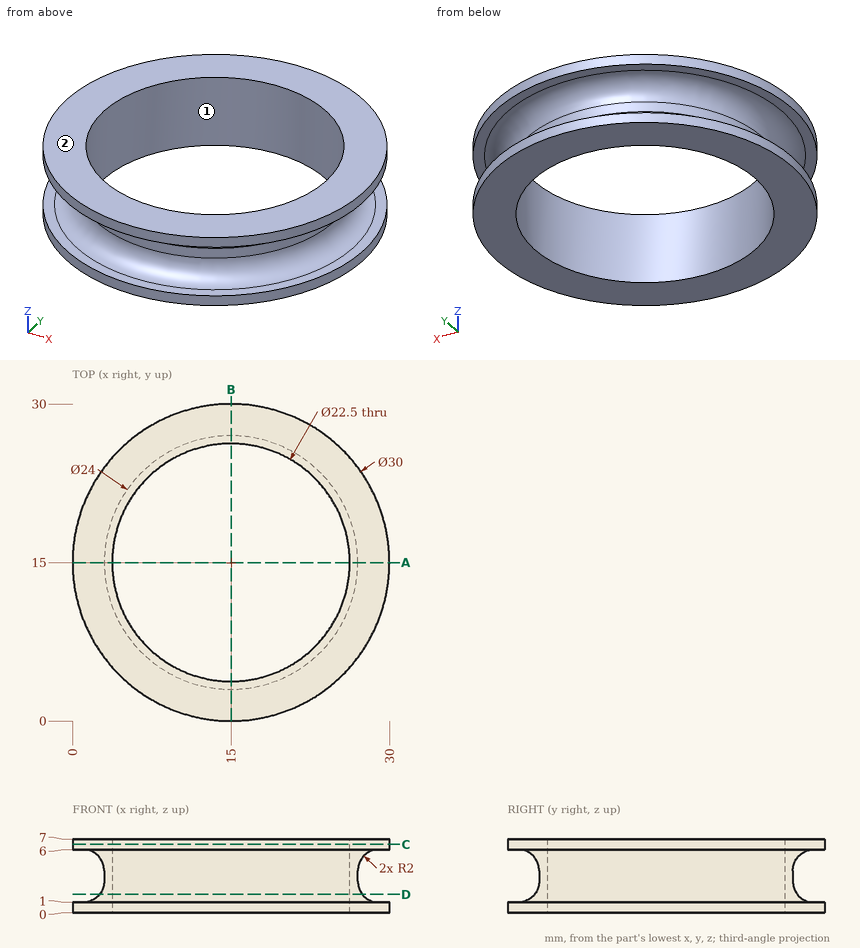
Design review of the part shown in the three views and the two pictorial views. Dimensions are in mm from the part's minimum x, y and z. Round coordinates to 2 decimals unless told otherwise and drop trailing zeros. Order: outer loops, then holes, each group sorted by start corner. A loop starts at its lowest first (then second) coordinate and runs counter-clockwise, first axis right, second up.
(1) Take a section at C-C, the plane z = 6.5. State the section outline as (x, y) points.
Working result:
outline: circle Ø30 at (15, 15); hole circle Ø22.5 at (15, 15)
(2) For P1, Ø4, axis at x = 13, z = 3.5, coming from the -Y side; P2, Ø10, axis at x = 21, y = 6.5, coming from the -Z side; P3, Ø2, axis at x = 21.5, y = 22, coming from the +Z side; P4, Ø1, axis at x = 17, z = 6, coming from the -Y side, all flat-tipped, find the tip position at first contact; note any pin that passes through.
Working result:
P1: stops at y = 2.46
P2: stops at z = 0
P3: passes through
P4: stops at y = 0.08
(3) Wall thickness on L1, parallel to Z at x = 1.5, y = 18; L2, parallel to Y at x = 15, z = 4; L3, parallel to X at y = 24.25, z = 5: over which ranges is each line inside the solid? List them lowest first.
Working result:
L1: z = 0 to 1.01, 5.99 to 7
L2: y = 3 to 3.75, 26.25 to 27
L3: x = 6.94 to 8.6, 21.4 to 23.06
(4) Mouldability with a two-part tool opening along Y and no side actions: class the marked faces 1 and 2 as released by +Y, released by -Y, zero draft, split by the parting line, or undercut.
Working result:
face 1: undercut
face 2: zero draft
(5) Take a section at A-A, the plane y = 15. State the section outline as (x, z) points.
Working result:
outline: (0, 0) - (3.75, 0) - (3.75, 7) - (0, 7) - (0, 6) - (1, 6) arc R2 cw to (3, 4) - (3, 3) arc R2 cw to (1, 1) - (0, 1) - close; (26.25, 0) - (30, 0) - (30, 1) - (29, 1) arc R2 cw to (27, 3) - (27, 4) arc R2 cw to (29, 6) - (30, 6) - (30, 7) - (26.25, 7) - close
(6) Take a section at D-D, the plane z = 1.75. State the section outline as (x, y) points.
Working result:
outline: circle Ø24.88 at (15, 15); hole circle Ø22.5 at (15, 15)
